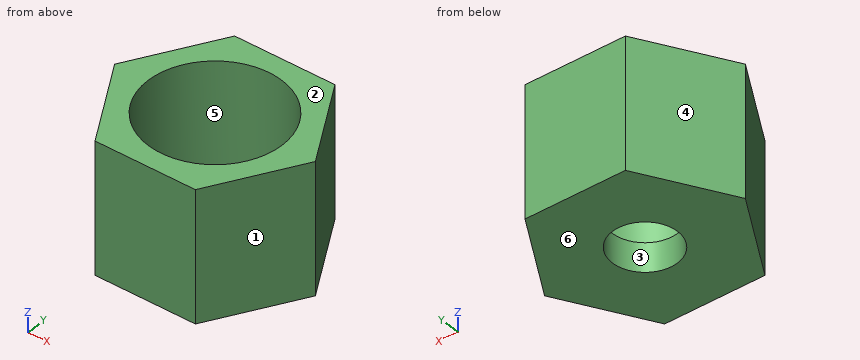
from build123d import *

# Parameters (mm, degrees)
BOSS_EXTRUDE1_DEPTH = 7.2009
SKETCH12_R          = 3.571875
CUT_EXTRUDE2_DEPTH  = 3.175
SKETCH11_R          = 7.34187
CUT_EXTRUDE3_DEPTH  = 11.2268


with BuildPart() as part:
    # Sketch1 → Boss-Extrude1 (new, symmetric)
    with BuildSketch(Plane.XY):
        Polygon((10.998522628, 0), (5.499261314, 9.525), (-5.499261314, 9.525), (-10.998522628, 0), (-5.499261314, -9.525), (5.499261314, -9.525), align=None)
    extrude(amount=BOSS_EXTRUDE1_DEPTH, both=True)

    # Sketch12 → Cut-Extrude2 (cut)
    with BuildSketch(Plane(origin=(0, 0, -7.2009), x_dir=(-1, 0, 0), z_dir=(0, 0, -1))):
        Circle(SKETCH12_R)
    extrude(amount=-CUT_EXTRUDE2_DEPTH, mode=Mode.SUBTRACT)

    # Sketch11 → Cut-Extrude3 (cut)
    with BuildSketch(Plane.XY.offset(7.2009)):
        Circle(SKETCH11_R)
    extrude(amount=-CUT_EXTRUDE3_DEPTH, mode=Mode.SUBTRACT)


solid = part.part
Check sheet for the modelled part. Datum: model origin and axes. Units: mm. Face numbers are marked on the shaded views. A direction names the side the tool comes from. Give positions to 0.01 mm unless a question says otherwise; leave off trailing zeros. Order: outer loops, then holes, each group sorted by start corner. A loop starts at its lowest first (then second) coordinate and runs counter-clockwise, first axis right, second up. Notation, with made-up numbers: M 85,37 L 124,37 A21 ccw 124,62 Z; hole C -10.5,40.5 d11. An arc over 180 degrees is marked long. Answer as CSV lines item,"result". Start each with the question number.
Item 1: Cross-section at D-D on z = -5. Enter the section's corners in (x, y) (3 decimals).
Item 2: Cross-section at B-B on z = 3.5. Enter the section's corners in (x, y) (3 decimals).
Item 3: Cross-section at A-A on x = 0. Enter the section's corners in (y, z) (3 decimals).
Item 4: Tool access check on the marked faces 5 and 6. Record the directions out of +Z, -Z, +X, -X, +Y, -Y that give a thin tool (end or side, any length) a straight path to the whole face; none if there is none.
Item 5: Mould release check, pull along Y, two halves, no side actions. Record for the marked faces 1, 2, 3 and 4: +Y half, -Y half, draft (parallel to the pull), parting line (faces both ways), or undercut.
Item 6: Cross-section at C-C on y = -1.25. Enter the section's corners in (x, z).
Item 7: Gauge pin test, flat ends, axial feed: P1, Ø4.5, axis at x = -2.5, y = 0, coming from the +Z side; P2, Ø1, axis at y = 4.5, z = -1, coming from the -X side; P3, Ø2, axis at y = -5.5, z = 0, coming from the -X side. Record the tip position at first contact, or that the pin passes through.
Item 8: Thickness scan on line 1 (Y direction, x = 0, z = -1.5) (3 decimals); line 2 (Z direction, x = 6, y = -3); line 3 (Y direction, x = -4.5, z = 4.25) (3 decimals). Record the ranges inside material, lowest first. Write a range as [from, to].
Established:
1,outline,"M -10.999,0 L -5.499,-9.525 L 5.499,-9.525 L 10.999,0 L 5.499,9.525 L -5.499,9.525 Z; hole C 0,0 d7.144"
2,outline,"M -10.999,0 L -5.499,-9.525 L 5.499,-9.525 L 10.999,0 L 5.499,9.525 L -5.499,9.525 Z; hole C 0,0 d14.684"
3,outline,"M -9.525,-7.201 L -3.572,-7.201 L -3.572,-4.026 L -7.342,-4.026 L -7.342,7.201 L -9.525,7.201 Z; M 3.572,-7.201 L 9.525,-7.201 L 9.525,7.201 L 7.342,7.201 L 7.342,-4.026 L 3.572,-4.026 Z"
4,face 5,"+Z"
4,face 6,"-Z, +X, -X, +Y, -Y"
5,face 1,"-Y half"
5,face 2,"draft"
5,face 3,"undercut"
5,face 4,"+Y half"
6,outline,"M -10.28,-7.2 L -3.35,-7.2 L -3.35,-4.03 L -7.23,-4.03 L -7.23,7.2 L -10.28,7.2 Z; M 3.35,-7.2 L 10.28,-7.2 L 10.28,7.2 L 7.23,7.2 L 7.23,-4.03 L 3.35,-4.03 Z"
7,P1,"stops at z = -4.03"
7,P2,"stops at x = -8.69"
7,P3,"stops at x = -8.4"
8,line 1,"y = [-9.525, -7.342], [7.342, 9.525]"
8,line 2,"z = [-7.2, -4.03]"
8,line 3,"y = [-9.525, -5.801], [5.801, 9.525]"
